The model under review builds one solid part; all positions refer to its coordinate system, in mm. Coordinates: 2 decimals unless noted, no trailing zeros. Write each loop counter-clockwise with the first axis right and the second up, starting at its lowest first coordinate (ties: lowest second). Pieces come first, ordered by that corner, then holes. Notation, with made-up numbers: M 84.25,53.5 L 117.25,53.5 A17 cw 117.25,74.5 Z; hole C 23,69.5 d9. An arc over 180 degrees is marked long. Answer as a JSON object with one key per item and string values.
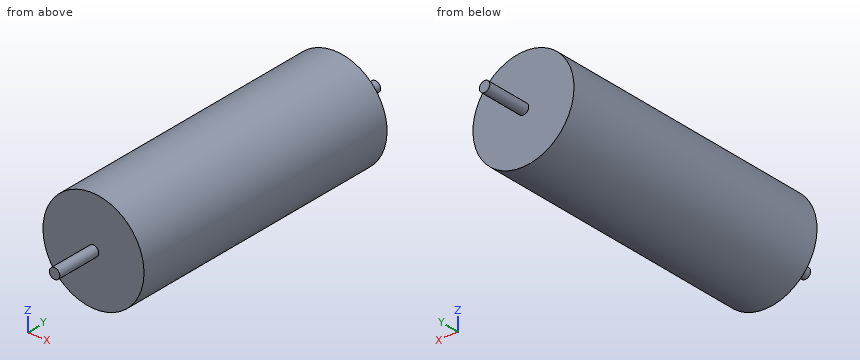
```python
from build123d import *

# Parameters (mm, degrees)
SKETCH1_R           = 114.3
BOSS_EXTRUDE1_DEPTH = 317.5
SKETCH2_R           = 11.811
BOSS_EXTRUDE2_DEPTH = 101.6
BOSS_EXTRUDE3_START = 101.6
SKETCH3_R           = 11.811
BOSS_EXTRUDE3_DEPTH = 101.6


with BuildPart() as part:
    # Sketch1 → Boss-Extrude1 (new, symmetric)
    with BuildSketch(Plane(origin=(0, 0, 0), x_dir=(1, 0, 0), z_dir=(0, 1, 0))):
        with Locations(Location((0, 0, 0), (0, 0, 90))):
            Circle(SKETCH1_R)
    extrude(amount=BOSS_EXTRUDE1_DEPTH, both=True)

    # Sketch2 → Boss-Extrude2 (add)
    with BuildSketch(Plane(origin=(0, 317.5, 0), x_dir=(1, 0, 0), z_dir=(0, 1, 0))):
        with Locations(Location((0, 0, 0), (0, 0, 270))):
            Circle(SKETCH2_R)
    extrude(amount=BOSS_EXTRUDE2_DEPTH)

    # Sketch3 → Boss-Extrude3 (add)
    with BuildSketch(Plane.XZ.offset(317.5).offset(BOSS_EXTRUDE3_START)):
        with Locations(Location((0, 0, 0), (0, 0, 90))):
            Circle(SKETCH3_R)
    extrude(amount=-BOSS_EXTRUDE3_DEPTH)


solid = part.part
```
(1) Add section C-C on y = 345.5. Give the boundary of the cut face in (x, z).
Results list:
{"outline": "C 0,0 d23.62"}
(2) For pin 1 Ø5 at (x, z) = (-19, 45) entering from +Y; pin 2 Ø4 at (y, z) = (-296.5, -7.5) entering from -X; pin 3 Ø8 at (x, z) = (54.5, 11.5) entering from -Y, all flat-tipped, find the tip position at first contact; note any pin that passes through.
Results list:
{"pin 1": "y = 317.5", "pin 2": "x = -114.17", "pin 3": "y = -317.5"}
(3) Add section A-A on z = 0. Give the boundary of the cut face in (x, y), and give its area (3 significant figures).
Results list:
{"outline": "M -114.3,-317.5 L -11.81,-317.5 L -11.81,-419.1 L 11.81,-419.1 L 11.81,-317.5 L 114.3,-317.5 L 114.3,317.5 L 11.81,317.5 L 11.81,419.1 L -11.81,419.1 L -11.81,317.5 L -114.3,317.5 Z", "area": "150,000 mm²"}
(4) Add section D-D on y = -4. Give the boundary of the cut face in (x, z), and give its area (3 significant figures).
Results list:
{"outline": "C 0,0 d228.6", "area": "41,000 mm²"}
(5) Wall thickness on line 1 along Y through (x, z) = (-39.5, -54.5); line 2 along Z through (x, y) = (2.5, -225.5); line 3 along X through (y, z) = (-127, 59.5): over which ranges is each line inside the solid? List them lowest first. Write a range as from..to.
Results list:
{"line 1": "-317.5..317.5", "line 2": "-114.27..114.27", "line 3": "-97.59..97.59"}
(6) Add section B-B on x = 0. Give the boundary of the cut face in (y, z).
Results list:
{"outline": "M -419.1,-11.81 L -317.5,-11.81 L -317.5,-114.3 L 317.5,-114.3 L 317.5,-11.81 L 419.1,-11.81 L 419.1,11.81 L 317.5,11.81 L 317.5,114.3 L -317.5,114.3 L -317.5,11.81 L -419.1,11.81 Z"}
